The drawing under review shows one solid part. Ordinate dimensions are in mm from its lowest x, y, z. A direction names the side the tool comes from. Coordinates: 2 decimals unless noted, no trailing zeros. Order: outer loops, then holes, each group sorted by start corner. A loop starts at its lowest first (then second) coordinate and runs counter-clockwise, first axis right, second up. Notation, with made-up numbers: M 86,88.25 L 133,88.25 A37 cw 133,125.25 Z; hole C 60.25,49.5 d7. An arc over 180 degrees is marked long. Answer as a JSON object with one key per item and string values.
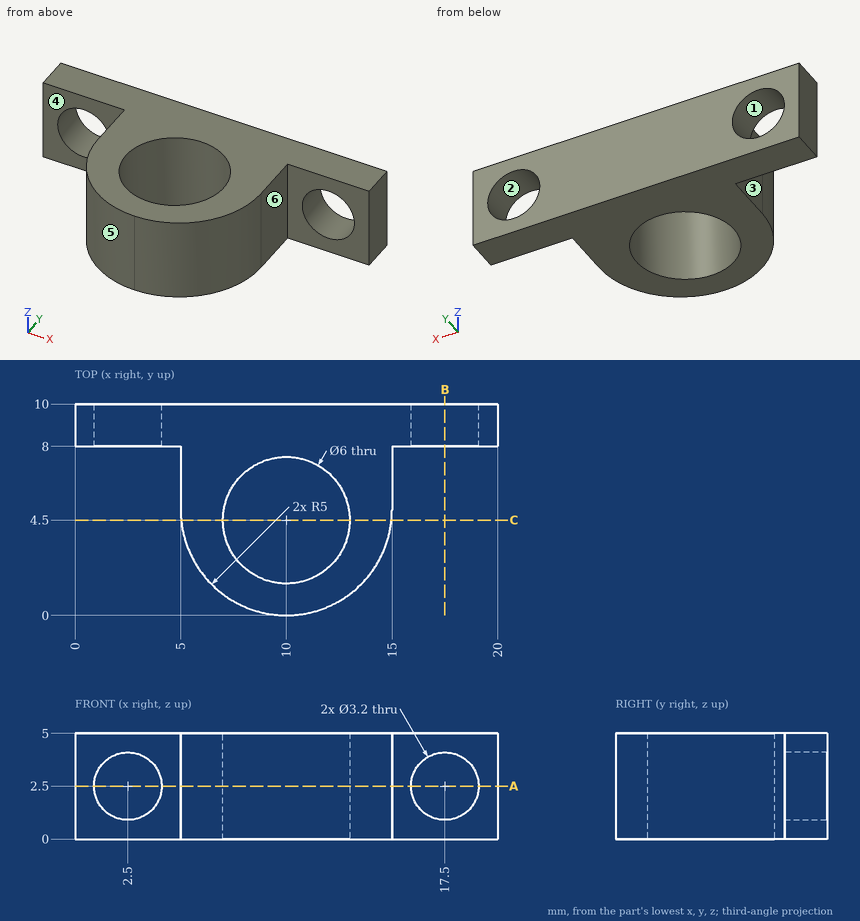
1) To check wall thickness, follow L1, parallel to X at y = 9.4, z = 2.5; L2, parallel to Y at x = 16, z = 3.9; L3, parallel to Y at x = 9.75, z = 4.6. State the ranges of each line that lie inside material, in increasing order.
Taken from the geometry:
{"L1": "x = 0 to 0.9, 4.1 to 15.9, 19.1 to 20", "L2": "y = 8 to 10", "L3": "y = 0.01 to 1.51, 7.49 to 10"}
2) Tool access review of the marked faces 5 and 6: name each direction out of +Z, -Z, +X, -X, +Y, -Y from which nothing blocks a thin tool from reaching the whole face with its end or side.
Taken from the geometry:
{"face 5": "+Z, -Z, -X, -Y", "face 6": "+Z, -Z, +X, -Y"}
3) Add section B-B (x = 17.5). State the section outline as (y, z) points.
Taken from the geometry:
{"outline": "M 8,0 L 10,0 L 10,0.9 L 8,0.9 Z; M 8,4.1 L 10,4.1 L 10,5 L 8,5 Z"}
4) Add section A-A (z = 2.5). Count the separate pieces of the cut face and the enclosed holes in it, and give its area (3 significant figures).
Taken from the geometry:
{"separate pieces": "3", "enclosed holes": "1", "area": "68.2 mm2"}
5) Add section C-C (y = 4.5). State the section outline as (x, z) points (3 decimals).
Taken from the geometry:
{"outline": "M 5.025,0 L 7,0 L 7,5 L 5.025,5 Z; M 13,0 L 14.975,0 L 14.975,5 L 13,5 Z"}
6) Insertion check: pin 1 Ø0.9 at (y, z) = (6.5, 1.5) entering from +X; pin 2 Ø1.9 at (x, z) = (2.5, 2.5) entering from +Y; pin 3 Ø1.5 at (x, z) = (1.5, 1.5) entering from -Y. Each pin has a flat end and moves straight along its axis. Give the tip position at first contact, or say it passes through.
Taken from the geometry:
{"pin 1": "stops at x = 15", "pin 2": "passes through", "pin 3": "stops at y = 8"}
7) Mouldability with a two-part tool opening along X and no side actions: class the marked faces 1, 2, 3 and 4 as released by +X, released by -X, zero draft, split by the parting line, or undercut.
Taken from the geometry:
{"face 1": "undercut", "face 2": "undercut", "face 3": "released by -X", "face 4": "zero draft"}
